Autodesk Inventor part; units mm, degrees
ref_plane "YZ Plane" through (0, 0, 0) normal (1, 0, 0) x (0, 1, 0)
ref_plane "XZ Plane" through (0, 0, 0) normal (0, 1, 0) x (-1, 0, 0)
ref_plane "XY Plane" through (0, 0, 0) normal (0, 0, 1) x (1, 0, 0)
sketch "Sketch1" plane through (0, 0, 0) normal (0, 1, 0) x (-1, 0, 0)
  line L0 (-12.7, 19.05) -> (12.7, 19.05)
  line L1 (12.7, 19.05) -> (12.7, -19.05)
  line L2 (12.7, -19.05) -> (-12.7, -19.05)
  line L3 (-12.7, -19.05) -> (-12.7, 19.05)
  line L4 (-12.7, 19.05) -> (12.7, -19.05) construction
  line L5 (12.7, 19.05) -> (-12.7, -19.05) construction
  circle A0 centre (0, 0) radius 2.286
  line L6 (12.7, 19.05) -> (-12.7, 19.05)
  line L7 (-12.7, 19.05) -> (-12.7, 34.29)
  line L8 (-12.7, 34.29) -> (12.7, 34.29)
  line L9 (12.7, 34.29) -> (12.7, 19.05)
  line L10 (-19.05, 19.05) -> (19.05, 19.05)
  line L11 (19.05, 19.05) -> (19.05, -19.05)
  line L12 (19.05, -19.05) -> (-19.05, -19.05)
  line L13 (-19.05, -19.05) -> (-19.05, 19.05)
  line L14 (-19.05, 19.05) -> (19.05, -19.05) construction
  line L15 (19.05, 19.05) -> (-19.05, -19.05) construction
  circle A1 centre (12.7, 0) radius 2.286
  circle A2 centre (-12.7, 0) radius 2.286
  line L16 (19.05, 19.05) -> (-19.05, 19.05)
  line L17 (-19.05, 19.05) -> (-19.05, 34.29)
  line L18 (-19.05, 34.29) -> (19.05, 34.29)
  line L19 (19.05, 34.29) -> (19.05, 19.05)
  circle A3 centre (0, 26.67) radius 2.286
  line L20 (-19.05, -19.05) -> (19.05, -19.05)
  line L21 (19.05, -19.05) -> (19.05, -20.32)
  line L22 (19.05, -20.32) -> (-19.05, -20.32)
  line L23 (-19.05, -20.32) -> (-19.05, -19.05)
  circle A4 centre (0, 0) radius 3.81
  circle A5 centre (-12.7, 0) radius 3.81
  circle A6 centre (12.7, 0) radius 3.81
  line L24 (0, 26.67) -> (-5.0038, 26.67)
  line L25 (-5.0038, 26.67) -> (0, 26.67)
  line L26 (0, 26.67) -> (5.0038, 26.67)
  circle A7 centre (5.0038, 26.67) radius 1.016
  circle A8 centre (-5.0038, 26.67) radius 1.016
  circle A9 centre (0, 19.05) radius 2.286
  circle A10 centre (-5.0038, 19.05) radius 1.016
  circle A11 centre (5.0038, 19.05) radius 1.016
  line L27 (-19.05, 26.67) -> (19.05, 26.67)
  point P0 (12.7, 34.29)
  dimension "d0" = 38.1
  dimension "d1" = 25.4
  dimension "d2" = 4.572
  dimension "d3" = 15.24
  dimension "d4" = 38.1
  dimension "d5" = 4.572
  dimension "d6" = 4.572
  dimension "d7" = 4.572
  dimension "d10" = 1.27
  dimension "d13" = 15.24
  dimension "d14" = 7.62
  dimension "d15" = 7.62
  dimension "d16" = 7.62
  dimension "d22" = 5.0038
  dimension "d23" = 5.0038
  dimension "d24" = 2.032
  dimension "d25" = 2.032
  dimension "d28" = 4.572
  dimension "d29" = 2.032
extrude "Extrusion1" add sketch "Sketch1" along normal blind 6.35 contours A11 L0 A9 A10 L7 L27 A8 L24 A3 L26 A7 L9 | A11 L0 | L0 A11 | L0 L1 A6 L2 L3 A5 A10 A9 A11 | L10 L11 L12 L1 A6 | L9 L27 L19 L10 | A6 L1 A1 | L1 A1 A6 | A7 L26 L27 | A10 L0 | L0 A10 | L12 L13 L10 L3 A5 | L7 L10 L17 L27 | A3 L24 L26 | A5 L3 A2 | L3 A2 A5 | L27 L24 A8 | A4 picked at (4.3363, 26.589) picked at (-1.5019, 26.4876) picked at (-5.6713, 26.589)
extrude "Extrusion2" add sketch "Sketch1" along normal blind 12.7 contours L21 L22 L23 L12 L2
extrude "Extrusion3" cut sketch "Sketch1" along normal blind 5.08 contours A6 L1 A1 | L1 A1 A6 | A5 L3 A2 | L3 A2 A5 | A4
sketch "Sketch2" plane through (0, 6.35, 0) normal (0, 1, 0) x (1, 0, 0)
  circle A0 centre (0, -26.67) radius 2.286
  circle A1 centre (0, -26.67) radius 3.81
  circle A2 centre (0, -19.0503) radius 3.81
  point P0 (0, 0)
  point P1 (0.035, -22.8602)
  point P2 (-0.035, -22.8602)
  dimension "d19" = 7.62
extrude "Extrusion4" cut sketch "Sketch2" against normal blind 5.08 contours A2
sketch "Sketch3" plane through (0, 0, 0) normal (0, -1, 0) x (1, 0, 0)
  point P0 (0, 0)
extrude "Extrusion5" cut sketch "Sketch1" along normal blind 4.445 contours A11 L0 | L0 A11 | A10 L0 | L0 A10
sketch "Sketch4" plane through (19.05, 0, -20.32) normal (0, 0, -1) x (-1, 0, 0)
  point P0 (19.05, 0)
sketch "Sketch5" plane through (-19.05, 6.35, -19.05) normal (0, 0, 1) x (1, 0, 0)
  line L0 (38.1, 6.35) -> (0, 6.35)
  line L1 (0, 6.35) -> (10.16, 6.35)
  line L2 (10.16, 6.35) -> (10.16, 0)
  line L3 (10.16, 0) -> (0, 0)
  line L4 (0, 0) -> (0, 6.35)
  line L5 (0, 0) -> (38.1, 0)
  line L6 (38.1, 6.35) -> (27.94, 6.35)
  line L7 (27.94, 6.35) -> (27.94, 0)
  line L8 (27.94, 0) -> (38.1, 0)
  line L9 (38.1, 0) -> (38.1, 6.35)
  point P0 (19.05, -6.35)
  dimension "d30" = 10.16
  dimension "d31" = 10.16
  dimension "d32" = 6.35
extrude "Extrusion6" cut sketch "Sketch5" against normal blind 25.4 contours L9 L5 L7 L0 | L2 L3 L4 L0
properties part number "BeamsplitterMounttoPolarisPinAdapterV3"
Work out the finished part from the listing and answer in its coordinate system (mm). A direction names the side the tool comes from. Coordinates: 2 decimals unless noted, no trailing zeros. Write each loop counter-clockwise with the first axis right and the second up, starting at its lowest first coordinate (ties: lowest second). Pieces come first, ordered by that corner, then holes.
Q1. Determine the mould class of faces 5 (the face through (-19.05, 3, 4)), 6 (the face through (0.5, 5.71, 2.23)), 7 (the face through (0, 12.7, -20)) for opening direction X: released by +X, released by -X, zero draft, split by the parting line, or undercut.
Q2. Find the intervals of material crossed by line 1 (Z direction, x = 0, y = 0.4); line 2 (X direction, y = 1.65, z = 19.05); line 3 (Z direction, x = -12.7, y = 2.55), in increasing order.
Q3. A cutting plane is placed at D-D, the plane y = 3. Give the vertices of the cut face in (x, z).
Q4. A cutting plane is placed at C-C, the plane x = 0. Give the vertices of the cut face in (y, z).
Q5. Each of these flat-tipped pins is pushed along its axis until it touches: pin 1 Ø3.5 at (x, z) = (12.7, 0) entering from -Y; pin 2 Ø6 at (x, z) = (0, 19.05) entering from +Y; pin 3 Ø2 at (x, z) = (-13.5, 16.5) entering from -Y; pin 4 Ø5 at (x, y) = (-1, 11) entering from +Z. Where does it stop, or does it pass through?
Q6. A cutting plane is placed at A-A, the plane x = -12.7. Give the vertices of the cut face in (y, z), then the cut area to 3 significant figures.
Q7. Which of the six approach directions +Z, -Z, +X, -X, +Y, -Y give full straight-line access (tool end or side, diameter ignored) to faces 1 (the face through (-8.89, 10, -20)), 2 (the face through (2, 1.27, 21)), 3 (the face through (-4, 0, 4)), 4 (the face through (-15.2, 5.08, 0.1))?
Q8. A cutting plane is placed at B-B, the plane z = 0. Give the vertices of the cut face in (x, y), then the cut area to 3 significant figures.
Findings below:
1. face 5: released by -X
1. face 6: undercut
1. face 7: zero draft
2. line 1: z = -20.32 to -3.81, 3.81 to 16.76, 21.34 to 26.67
2. line 2: x = -19.05 to -6.02, -3.99 to -3.81, 3.81 to 3.99, 6.02 to 19.05
2. line 3: z = -20.32 to -3.81, 3.81 to 26.67
3. outline: (-19.05, -20.32) - (19.05, -20.32) - (19.05, 26.67) - (-19.05, 26.67) - close; hole circle Ø7.62 at (-12.7, 0); hole circle Ø2.03 at (-5, 19.05); hole circle Ø7.62 at (0, 0); hole circle Ø7.62 at (0, 19.05); hole circle Ø2.03 at (5, 19.05); hole circle Ø7.62 at (12.7, 0)
4. outline: (0, -20.32) - (12.7, -20.32) - (12.7, -19.05) - (6.35, -19.05) - (6.35, -2.29) - (5.08, -2.29) - (5.08, -3.81) - (0, -3.81) - close; (0, 3.81) - (5.08, 3.81) - (5.08, 2.29) - (6.35, 2.29) - (6.35, 15.24) - (1.27, 15.24) - (1.27, 16.76) - (0, 16.76) - close; (0, 21.34) - (1.27, 21.34) - (1.27, 22.86) - (6.35, 22.86) - (6.35, 26.67) - (0, 26.67) - close
5. pin 1: passes through
5. pin 2: stops at y = 1.27
5. pin 3: stops at y = 0
5. pin 4: stops at z = -19.05
6. outline: (0, -20.32) - (6.35, -20.32) - (6.35, -2.29) - (5.08, -2.29) - (5.08, -3.81) - (0, -3.81) - close; (0, 3.81) - (5.08, 3.81) - (5.08, 2.29) - (6.35, 2.29) - (6.35, 26.67) - (0, 26.67) - close
6. area: 254 mm2
7. face 1: +Z, -Z, -X, +Y
7. face 2: +Y
7. face 3: +Z, -Z, +X, -X, -Y
7. face 4: -Y
8. outline: (-19.05, 0) - (-16.51, 0) - (-16.51, 5.08) - (-14.99, 5.08) - (-14.99, 6.35) - (-19.05, 6.35) - close; (-10.41, 5.08) - (-8.89, 5.08) - (-8.89, 0) - (-3.81, 0) - (-3.81, 5.08) - (-2.29, 5.08) - (-2.29, 6.35) - (-10.41, 6.35) - close; (2.29, 5.08) - (3.81, 5.08) - (3.81, 0) - (8.89, 0) - (8.89, 5.08) - (10.41, 5.08) - (10.41, 6.35) - (2.29, 6.35) - close; (14.99, 5.08) - (16.51, 5.08) - (16.51, 0) - (19.05, 0) - (19.05, 6.35) - (14.99, 6.35) - close
8. area: 108 mm2
